Model file for the job. Use its own axes, mm. Face numbers are marked on the shaded views. A direction names the side the tool comes from. Coordinates: 2 decimals unless noted, no trailing zeros. Write each loop counter-clockwise with the first axis right and the second up, starting at its lowest first coordinate (ties: lowest second). Pieces come first, ordered by that corner, then holes. Notation, with made-up numbers: M -30.75,-5.5 L -3.75,-5.5 A22 ccw -3.75,20.5 Z; hole C 64,-39 d7. An arc over 180 degrees is marked long. Put each result on its own line as item: value. Start each with the question number.
Q1. Cut at A-A (x = 21). Write the cut outline in (y, z).
Q2. Drill centre lines: line 1 along X through (y, z) = (1.25, -26); line 2 along X through (y, z) = (4.55, -31.5); line 3 along X through (y, z) = (3, -37.5). Where is each one in solid material? Low to high.
Q3. Drop flat-ended pins along their axis: pin 1 (5 mm diameter, centred on x = 44.19, z = -48.34, fed in from +Y); pin 2 (2.5 mm diameter, centred on x = 4.86, z = -48.34, fed in from +Y); pin 3 (3 mm diameter, centred on x = 35, y = 2.5, fed in from +Z); pin 4 (3 mm diameter, centred on x = 1, y = 2.5, fed in from -Z). Give the stop position or say it passes through.
Q4. Pull direction X, two halves, no side cores. Call the marked faces 1, 2 and 3: pulls with the +X half, pulls with the -X half, needs draft (parallel to the pull), parting line crosses it, or undercut.
Q5. Cut at B-B (y = 0.85). Give the number of separate pieces and of enclosed holes in the cut face, then the cut area to 3 significant figures.
Q6. Cut at C-C (x = 32.5). Write the cut outline in (y, z).
Q7. Which spindle directions (+Z, -Z, +X, -X, +Y, -Y) get a long thin tool onto all of the face, cutting with end or side? Do the marked faces 4 and 5. Say none if no direction does.
Q8. Cut at D-D (z = -53). Write the cut outline in (x, y).
```python
from build123d import *

# Parameters (mm, degrees)
BOSS_EXTRUDE2_DEPTH = 5
SKETCH2_R           = 1.5
CUT_EXTRUDE1_DEPTH  = 15


with BuildPart() as part:
    # Sketch1 → Boss-Extrude2 (new body)
    with BuildSketch(Plane(origin=(0, 0, 0), x_dir=(1, 0, 0), z_dir=(0, 1, 0))):
        with BuildLine():
            Line((1.569728042, 52.040332943), (15.651301799, 56.559771658))
            Line((15.651301799, 56.559771658), (39.856221019, 56.858644564))
            Line((39.856221019, 56.858644564), (53.599377939, 46.535137731))
            Line((53.599377939, 46.535137731), (57.29105631, 36.738583337))
            Line((57.29105631, 36.738583337), (56.448543902, 24.628756692))
            Line((56.448543902, 24.628756692), (46.012568554, 15.301947443))
            Line((46.012568554, 15.301947443), (36.148543795, 16.282769063))
            ThreePointArc((36.148543795, 16.282769063), (30.610071526, 20.095537749), (24.030369651, 21.480963085))
            ThreePointArc((24.030369651, 21.480963085), (10.748506444, 14.399234116), (6.364349479, 0))
            ThreePointArc((6.364349479, 0), (5.689983794, -1.843684392), (4.107122834, -3.004930446))
            Line((4.107122834, -3.004930446), (-2.771373889, -2.820272816))
            ThreePointArc((-2.771373889, -2.820272816), (-3.97819548, -2.210628496), (-4.733361209, -1.089107533))
            Line((-4.733361209, -1.089107533), (-9.544633948, 27.008719122))
            Line((-9.544633948, 27.008719122), (-7.668325905, 42.684434119))
            Line((-7.668325905, 42.684434119), (1.569728042, 52.040332943))
        make_face()
        with BuildLine():
            Line((1.036932163, 38.743694932), (-0.578535299, 23.81135118))
            Line((-0.578535299, 23.81135118), (6.824389086, 23.010459929))
            ThreePointArc((6.824389086, 23.010459929), (22.804886304, 29.960497456), (39.395602183, 24.628756692))
            Line((39.395602183, 24.628756692), (43.340115732, 24.258511233))
            Line((43.340115732, 24.258511233), (48.476214586, 28.525175745))
            Line((48.476214586, 28.525175745), (49.056861781, 34.804762264))
            Line((49.056861781, 34.804762264), (46.61935743, 41.212721012))
            Line((46.61935743, 41.212721012), (37.197706882, 48.312593262))
            Line((37.197706882, 48.312593262), (17.555979737, 47.985159309))
            Line((17.555979737, 47.985159309), (6.642360366, 44.349123135))
            Line((6.642360366, 44.349123135), (1.036932163, 38.743694932))
        make_face(mode=Mode.SUBTRACT)
    extrude(amount=BOSS_EXTRUDE2_DEPTH)

    # Sketch2 → Cut-Extrude1 (cut)
    with BuildSketch(Plane(origin=(0, 5, 0), x_dir=(1, 0, 0), z_dir=(0, 1, 0))):
        with Locations((44.194472597, 48.335123533)):
            Circle(SKETCH2_R)
        Circle(SKETCH2_R)
        with Locations((4.859386625, 48.335123533)):
            Circle(SKETCH2_R)
    extrude(amount=-CUT_EXTRUDE1_DEPTH, mode=Mode.SUBTRACT)


solid = part.part
```
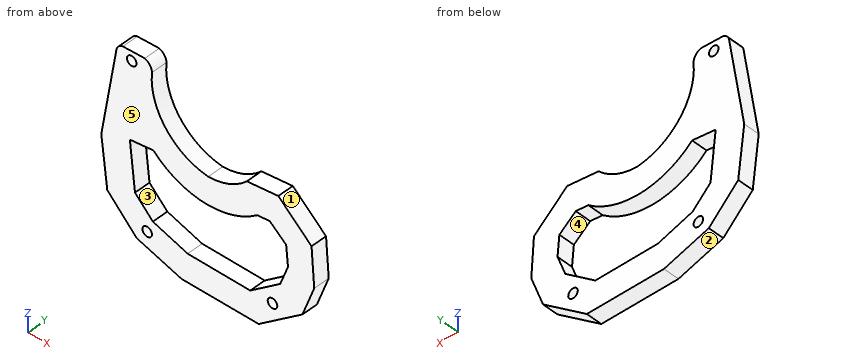
Computed values:
1. outline: M 0,-56.63 L 5,-56.63 L 5,-48.04 L 0,-48.04 Z; M 0,-29.8 L 5,-29.8 L 5,-20.94 L 0,-20.94 Z
2. line 1: -9.37 to -0.34, 10.57 to 37.49, 45.44 to 56.54
2. line 2: -9.01 to 0.25, 48.75 to 56.93
2. line 3: -8.29 to 0.9, 48.03 to 57
3. pin 1: y = 5
3. pin 2: through
3. pin 3: z = -16.25
3. pin 4: z = -52.34
4. face 1: pulls with the +X half
4. face 2: pulls with the -X half
4. face 3: undercut
5. separate pieces: 1
5. enclosed holes: 4
5. area: 1,610 mm2
6. outline: M 0,-56.77 L 5,-56.77 L 5,-48.23 L 0,-48.23 Z; M 0,-28.49 L 5,-28.49 L 5,-19.14 L 0,-19.14 Z
7. face 4: +Y, -Y
7. face 5: +Z, -Z, +X, -X, -Y
8. outline: M 4.56,0 L 44.99,0 L 44.99,5 L 4.56,5 Z
